Input: part model. Units: mm. Frame: model coordinates. A direction names the side the tool comes from. Round coordinates to 2 decimals unless told otherwise and drop trailing zeros. Write each loop counter-clockwise with the first axis right and the second up, starting at its lowest first coordinate (ties: lowest second). Pieces come first, ordered by that corner, then holes. Notation, with made-up numbers: (0, 4.5) -> (53, 4.5) arc R22 cw to (53, 23.5) -> close; hole circle Ø7 at (83, 21.25). An arc over 180 degrees is marked (long way). Use CSV: the item, a comma, the result in double quotes.
Autodesk Inventor part; units mm, degrees
ref_plane "Work Plane1" through (0, 3, 0) normal (0, 1, 0) x (-1, 0, 0)
ref_plane "YZ Plane" through (0, 0, 0) normal (1, 0, 0) x (0, 1, 0)
ref_plane "XY Plane" through (0, 0, 0) normal (0, 0, 1) x (1, 0, 0)
sketch "Sketch1" plane through (0, 0, 0) normal (0, 1, 0) x (-1, 0, 0)
  line L0 (-51.65, 23.5) -> (51.65, 23.5)
  line L1 (54.65, 20.5) -> (54.65, -20.5)
  line L2 (51.65, -23.5) -> (-51.65, -23.5)
  line L3 (-54.65, -20.5) -> (-54.65, 20.5)
  circle A0 centre (-47.65, 16.5) radius 2.25
  circle A1 centre (47.65, 16.5) radius 2.25
  circle A2 centre (-47.65, 16.5) radius 26.75 construction
  circle A3 centre (-10.7, 16.5) radius 2.25
  circle A4 centre (-10.7, 16.5) radius 11.2 construction
  line L4 (-21.9, 16.5) -> (-21.9, 6.8604)
  line L5 (-20.9, 16.5) -> (-20.9, 6.8604)
  circle A5 centre (10.7, 16.5) radius 2.25
  circle A6 centre (10.7, 16.5) radius 11.2 construction
  line L6 (-0.5, 16.5) -> (-0.5, 5.694)
  line L7 (0.5, 16.5) -> (0.5, 5.694)
  circle A7 centre (47.65, 16.5) radius 26.75 construction
  line L8 (20.9, 16.5) -> (20.9, 5.8426)
  line L9 (21.9, 16.5) -> (21.9, 5.8426)
  arc A8 (-51.65, 23.5) -> (-54.65, 20.5) centre (-51.65, 20.5) ccw
  arc A9 (-54.65, -20.5) -> (-51.65, -23.5) centre (-51.65, -20.5) ccw
  arc A10 (54.65, 20.5) -> (51.65, 23.5) centre (51.65, 20.5) ccw
  arc A11 (51.65, -23.5) -> (54.65, -20.5) centre (51.65, -20.5) ccw
  line L10 (-84.9483, 16.5) -> (77.5332, 16.5) construction
  line L11 (-54.65, 0) -> (54.65, 0)
  line L12 (10.7, 30.5) -> (10.7, -33.5) construction
  circle A12 centre (10.7, -16.5) radius 2.25
  line L13 (5, -8.5) -> (18, -8.5) construction
  line L14 (3.7, -4.5) -> (3.7, -33.5) construction
  line L15 (-6.3, -4.5) -> (-6.3, -33.5) construction
  line L16 (-1.3, -33.5) -> (-1.3, -4.5) construction
  circle A13 centre (-1.3, -38.9) radius 2.25
  circle A14 centre (-1.3, -8.5) radius 2.25
  line L17 (-17.7373, -23.5) -> (14.2274, -23.5)
  line L18 (14.2274, -23.5) -> (14.2274, -45.3565)
  line L19 (14.2274, -45.3565) -> (-17.7373, -45.3565)
  line L20 (-17.7373, -45.3565) -> (-17.7373, -23.5)
  line L21 (-40.65, 5) -> (-30.65, 5)
  line L22 (-30.65, 5) -> (-30.65, -5)
  line L23 (-30.65, -5) -> (-40.65, -5)
  line L24 (-40.65, -5) -> (-40.65, 5)
  line L25 (-42.65, -7) -> (-28.65, -7)
  line L26 (-28.65, -7) -> (-28.65, 7)
  line L27 (-28.65, 7) -> (-42.65, 7)
  line L28 (-42.65, 7) -> (-42.65, -7)
  point P0 (0, 0)
  point P1 (-54.65, 23.5)
  point P2 (-54.65, -23.5)
  point P3 (0, 23.5)
  point P4 (-35.65, 5)
  point P5 (-30.65, 0)
  dimension "d5" = 53.5
  dimension "d12" = 53.5
  dimension "d1" = 4.5
  dimension "d2" = 7
  dimension "d3" = 4.5
  dimension "d4" = 7
  dimension "d6" = 4.5
  dimension "d7" = 22.4
  dimension "d8" = 1
  dimension "d9" = 4.5
  dimension "d10" = 22.4
  dimension "d11" = 1
  dimension "d13" = 1
  dimension "d14" = 3
  dimension "d23" = 16.5
  dimension "d24" = 7
  dimension "d27" = 8
  dimension "d28" = 7
  dimension "d29" = 10
  dimension "d30" = 5
  dimension "d31" = 4.5
  dimension "d32" = 4.5
  dimension "d33" = 30.4
  dimension "d38" = 0
  dimension "d40" = 10
  dimension "d41" = 10
  dimension "d43" = 2
  dimension "d47" = 12
ref_plane "Work Plane1" through (0, 3, 0) normal (0, 1, 0) x (-1, 0, 0)
sketch "Sketch3" plane through (0, 3, 0) normal (0, 1, 0) x (-1, 0, 0)
  circle A0 centre (-10.7, -16.5) radius 2.25
  circle A1 centre (10.7, -16.5) radius 2.25
  circle A2 centre (10.7, 16.5) radius 2.25
  circle A3 centre (-10.7, 16.5) radius 2.25
  line L0 (-17.7, -23.5) -> (17.7, -23.5)
  line L1 (17.7, 23.5) -> (-17.7, 23.5)
  line L2 (-17.7, 23.5) -> (-17.7, -23.5)
  line L3 (17.7, 23.5) -> (17.7, -23.5)
  line L4 (-40, 23.5) -> (40, 23.5)
  line L5 (40, 23.5) -> (40, 63.5)
  line L6 (40, 63.5) -> (-40, 63.5)
  line L7 (-40, 63.5) -> (-40, 23.5)
  line L8 (-20, 63.5) -> (20, 63.5)
  line L9 (20, 63.5) -> (20, 40)
  line L10 (20, 40) -> (-20, 40)
  line L11 (-20, 40) -> (-20, 63.5)
  line L12 (0, 0) -> (0, -39.7707) construction
  line L13 (0, 40) -> (0, 63.5) construction
  line L14 (-40, 23.5) -> (-40, 9.5)
  line L15 (-40, 9.5) -> (40, 9.5)
  line L16 (40, 9.5) -> (40, 23.5)
  circle A4 centre (-27, 58.5) radius 2.25
  line L17 (-20, 40) -> (-34, 40)
  line L18 (-34, 40) -> (-34, 63.5)
  line L19 (-34, 63.5) -> (-20, 63.5)
  line L20 (-20, 63.5) -> (-20, 40)
  circle A5 centre (-27, 45) radius 2.25
  line L21 (-20, 38) -> (-34, 38)
  line L22 (-36, 38) -> (-36, 63.5)
  line L23 (-20, 38) -> (-20, 40)
  line L24 (-36, 63.5) -> (-34, 63.5)
  line L25 (20, 40) -> (20, 38)
  line L26 (-34, 38) -> (-36, 38)
  line L27 (-20, 38) -> (20, 38)
  line L28 (-36, 54.8338) -> (-34, 54.8338)
  point P0 (0, 63.5)
  point P1 (0, 23.5)
  point P2 (-27, 63.5)
  dimension "d67" = 7
  dimension "d73" = 7
  dimension "d74" = 7
  dimension "d84" = 7
  dimension "d86" = 7
  dimension "d87" = 40
  dimension "d88" = 80
  dimension "d91" = 40
  dimension "d92" = 23.5
  dimension "d96" = 4.5
  dimension "d97" = 7
  dimension "d98" = 4.5
  dimension "d99" = 7
  dimension "d100" = 5
  dimension "d101" = 4.5
  dimension "d102" = 7
  dimension "d103" = 5
  dimension "d104" = 2
extrude "Extrusion8" add sketch "Sketch3" along normal blind 3 contours L2 L15 L3 L0 | L15 L14 L4 L2 | L2 L1 L3 L15 | L3 L4 L16 L15 | L4 L7 L6 L22 L26 L21 L27 L25 L9 L5 L1 | L6 L18 L28 L22 | L9 L10 L11 L6 | L6 L11 L17 L18 | L28 L18 L17 L23 L21 L26 L22 | L25 L27 L23 L10 | A4 | A5
extrude "Extrusion9" cut sketch "Sketch3" along normal blind 1 contours L28 L18 L17 L23 L21 L26 L22 | L25 L27 L23 L10
extrude "Extrusion10" cut sketch "Sketch3" along normal blind 10 contours A4 | A5
mirror "Mirror4" about plane through (0, 0, 0) normal (1, 0, 0) of "Extrusion9", "Extrusion10"
fillet "Fillet3" radius 10 4 edges at (-40, 4.5, 9.5) (-17.7, 4.5, 9.5) (17.7, 4.5, 9.5) (40, 4.5, 9.5)
fillet "Fillet4" radius 4 4 edges at (-40, 4.5, 63.5) (40, 4.5, 63.5) (-17.7, 4.5, -23.5) (17.7, 4.5, -23.5)
properties part number "OuterBar"
Item 1: Section query C-C on y = 5.25. Give the number of separate pieces and of enclosed holes in the cut face, plus the area to 3 significant figures.
Worked answers:
separate pieces,"1"
enclosed holes,"8"
area,"5,350 mm²"
Item 2: Set-up query: faces 1 (the face through (-17.7, 4, -10)), 2 (the face through (-10.212, 4.479, 18.696)). Return all of +Z, -Z, +X, -X, +Y, -Y with unobstructed straight access to the full face (end or side cutting, diameter ignored); none if empty.
Worked answers:
face 1,"-Z, -X, +Y, -Y"
face 2,"+Y, -Y"
Item 3: Section query B-B on x = 10.7. Return the cut outline in (y, z).
Worked answers:
outline,"(3, -23.5) -> (6, -23.5) -> (6, -18.75) -> (3, -18.75) -> close; (3, -14.25) -> (6, -14.25) -> (6, 14.25) -> (3, 14.25) -> close; (3, 18.75) -> (6, 18.75) -> (6, 63.5) -> (3, 63.5) -> (3, 40) -> (4, 40) -> (4, 38) -> (3, 38) -> close"
Item 4: Line query: line 1 (Z direction, x = 10.7, y = 5.1); line 2 (X direction, y = 4.95, z = 17); line 3 (Z direction, x = -27, y = 3.8). Output: solid intervals per line, ascending.
Worked answers:
line 1,"z = -23.5 to -18.75, -14.25 to 14.25, 18.75 to 63.5"
line 2,"x = -39.68 to -12.89, -8.51 to 8.51, 12.89 to 39.68"
line 3,"z = 9.48 to 38, 40 to 42.75, 47.25 to 56.25, 60.75 to 63.5"
Item 5: First-contact query: pin 1 Ø0.9 at (y, z) = (4, -6) entering from -X. Flat tip, straight axial feed; report the tip coordinate or a pass-through.
Worked answers:
pin 1,"stops at x = -17.7"
Item 6: Pull-direction query (X, two-part tool) for faces 3 (the face through (-36.99, 4.52, 12.35)), 4 (the face through (-10.212, 4.479, -14.304)), 5 (the face through (37.15, 4.52, 12.51)); classes: +X half, -X half, draft (parallel to the pull), parting line (faces both ways), or undercut.
Worked answers:
face 3,"-X half"
face 4,"undercut"
face 5,"+X half"
Item 7: Section query D-D on z = 58.5. Return the cut outline in (x, y).
Worked answers:
outline,"(-40, 3) -> (-29.25, 3) -> (-29.25, 6) -> (-40, 6) -> close; (-24.75, 3) -> (24.75, 3) -> (24.75, 6) -> (-24.75, 6) -> close; (29.25, 3) -> (40, 3) -> (40, 6) -> (29.25, 6) -> close"
Item 8: Section query A-A on z = 45. Return the cut outline in (x, y).
Worked answers:
outline,"(-40, 3) -> (-36, 3) -> (-36, 4) -> (-34, 4) -> (-34, 3) -> (-29.25, 3) -> (-29.25, 6) -> (-40, 6) -> close; (-24.75, 3) -> (24.75, 3) -> (24.75, 6) -> (-24.75, 6) -> close; (29.25, 3) -> (34, 3) -> (34, 4) -> (36, 4) -> (36, 3) -> (40, 3) -> (40, 6) -> (29.25, 6) -> close"
